```python
from build123d import *

# Parameters (mm, degrees)
SKETCH007_W            = 184
SKETCH007_H            = 240
PAD006_DEPTH           = 1.5
SKETCH009_W            = 5
SKETCH009_H            = 240
PAD007_DEPTH           = 43.5
PAD008_DEPTH           = 179
SKETCH008_R            = 2.6
POCKET_DEPTH           = 45.001
LINEARPATTERN002_COUNT = 4
LINEARPATTERN002_PITCH = 60
SKETCH011_R            = 2.6
POCKET001_DEPTH        = 45.001
LINEARPATTERN003_COUNT = 3
LINEARPATTERN003_PITCH = 60
SKETCH012_R            = 1.55
POCKET002_DEPTH        = 45.001
FILLET003_R            = 1


with BuildPart() as part:
    # Sketch007 (on XY_Plane001 of Origin002) → Pad006 (new body)
    with BuildSketch(Plane.XY):
        with Locations((292, 120)):
            Rectangle(SKETCH007_W, SKETCH007_H)
    extrude(amount=PAD006_DEPTH)

    # Sketch009 (on Face4 of Pad006) → Pad007 (join)
    with BuildSketch(Plane.XY.offset(1.5)):
        with Locations((381.5, 120)):
            Rectangle(SKETCH009_W, SKETCH009_H)
    extrude(amount=PAD007_DEPTH)

    # Sketch010 (on Face4 of Pad007) → Pad008 (join)
    with BuildSketch(Plane(origin=(379, 0, 0), x_dir=(0, -1, 0), z_dir=(-1, 0, 0))):
        Polygon((0, 1.5), (0, 4.5), (-2, 4.5), (-5, 1.5), align=None)
    extrude(amount=PAD008_DEPTH)

    # Sketch008 (on XY_Plane001 of Origin002) → Pocket (cut, through all)
    with BuildSketch(Plane.XY):
        with Locations((202, 10)):
            Circle(SKETCH008_R)
    pocket = extrude(amount=POCKET_DEPTH, mode=Mode.SUBTRACT)

    # LinearPattern002: Pocket ×4
    with Locations(*[(0, i * LINEARPATTERN002_PITCH, 0) for i in range(1, LINEARPATTERN002_COUNT)]):
        add(pocket, mode=Mode.SUBTRACT)

    # Sketch011 (on XY_Plane001 of Origin002) → Pocket001 (cut, through all)
    with BuildSketch(Plane.XY):
        with Locations((210, 238)):
            Circle(SKETCH011_R)
    pocket001 = extrude(amount=POCKET001_DEPTH, mode=Mode.SUBTRACT)

    # LinearPattern003: Pocket001 ×3
    with Locations(*[(i * LINEARPATTERN003_PITCH, 0, 0) for i in range(1, LINEARPATTERN003_COUNT)]):
        add(pocket001, mode=Mode.SUBTRACT)

    # Sketch012 (on XY_Plane001 of Origin002) → Pocket002 (cut, through all)
    with BuildSketch(Plane.XY):
        with Locations((381.5, 239)):
            Circle(SKETCH012_R)
    extrude(amount=POCKET002_DEPTH, mode=Mode.SUBTRACT)

    # Fillet003
    fillet003_edges = [part.edges().sort_by_distance(p)[0] for p in [
        (381.5, 0, 45),
        (379, 120, 45),
        (384, 120, 45),
        (384, 0, 22.5),
        (379, 0, 24.75),
    ]]
    fillet(fillet003_edges, radius=FILLET003_R)


solid = part.part
```
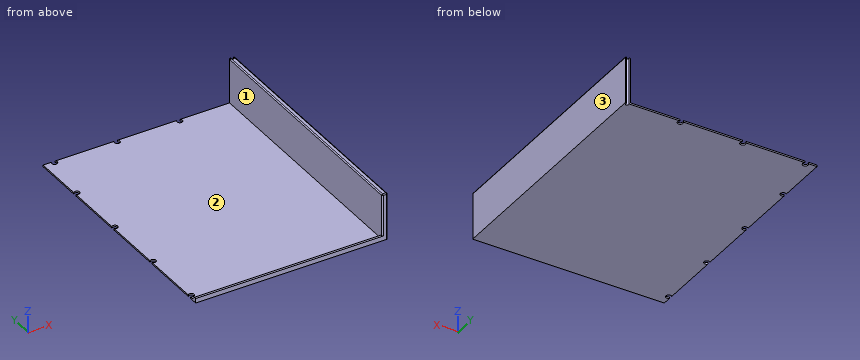
Can you work these out from the model? Positions are in its coordinate system, mm. Face numbers are marked on the shaded views. Round coordinates to 2 decimals unless told otherwise and drop trailing zeros. Loops run counter-clockwise (first coordinate to the right, second up) from the corner with the lowest first, then second, coordinate; pieces in that order, holes last. Notation, with made-up numbers: (-9.5, -30.5) -> (26.5, -30.5) arc R9 cw to (26.5, -20.5) -> close; hole circle Ø7 at (84, 58.5). An arc over 180 degrees is marked (long way). One line per item, written item: value. Start each with the question number.
1. If we section it at B-B, the plane z = 32: Write out the boundary of the cut face in (x, y).
2. For pin 1 (6 mm diameter, centred on x = 210, y = 238, fed in from +Z); pin 2 (4 mm diameter, centred on y = 173.5, z = 16.5, fed in from -X); pin 3 (1.6 mm diameter, centred on x = 322.5, y = 1.5, fed in from +Z), each with a flat end and sliding along its axis, tell me the tip position at first contact or that it passes through.
3. If I drill on probe 1 along X at (y, z) = (238, 1); probe 2 along Y at (x, z) = (202, 1); probe 3 along X at (y, z) = (239, 23), over which ranges is the centre line in solid material (lowest first)?
4. If we section it at A-A, the plane y = 111: Write out the boundary of the cut face in (x, z), then the cut area to 3 significant figures.
5. If we mould it in two halves opening along X, with no side actions, what happens to the marked faces 1, 2 and 3? For each: pulls with the +X half, pulls with the -X half, needs draft (parallel to the pull), parting line crosses it, or undercut.
6. If we section it at C-C, the plane x = 260: Write out the boundary of the cut face in (y, z).
Calculated:
1. outline: (379, 1) arc R1 ccw to (380, 0) -> (383, 0) arc R1 ccw to (384, 1) -> (384, 240) -> (382.68, 240) arc R1.55 cw (long way) to (380.32, 240) -> (379, 240) -> close
2. pin 1: stops at z = 1.5
2. pin 2: stops at x = 379
2. pin 3: stops at z = 4.5
3. probe 1: x = 200 to 207.4, 212.6 to 267.4, 272.6 to 327.4, 332.6 to 380.32, 382.68 to 384
3. probe 2: y = 0 to 7.4, 12.6 to 67.4, 72.6 to 127.4, 132.6 to 187.4, 192.6 to 240
3. probe 3: x = 379 to 379.95, 383.05 to 384
4. outline: (200, 0) -> (384, 0) -> (384, 44) arc R1 ccw to (383, 45) -> (380, 45) arc R1 ccw to (379, 44) -> (379, 1.5) -> (200, 1.5) -> close
4. area: 493 mm²
5. face 1: pulls with the -X half
5. face 2: needs draft
5. face 3: pulls with the +X half
6. outline: (0, 0) -> (240, 0) -> (240, 1.5) -> (5, 1.5) -> (2, 4.5) -> (0, 4.5) -> close
